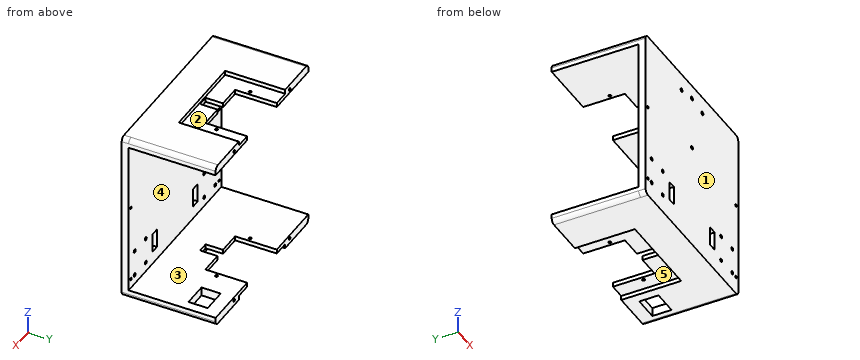
from build123d import *

# Parameters (mm, degrees)
SKETCH_1_W          = 200
SKETCH_1_H          = 200
SKETCH_1_R          = 2.05
SKETCH_1_R_2        = 1.6
SKETCH_1_R_3        = 2.1
SKETCH_1_W_2        = 10
SKETCH_1_H_2        = 22
EXTRUDE_1_DEPTH     = 8
FILLET_1_R          = 5
FILLET_2_R          = 5
FILLET_3_R          = 5
FILLET_4_R          = 5
SKETCH_2_W          = 200
SKETCH_2_H          = 10
EXTRUDE_2_DEPTH     = 100
FILLET_5_R          = 5
FILLET_6_R          = 5
FILLET_7_R          = 5
FILLET_8_R          = 5
SKETCH_3_R          = 1.6
CUT_EXTRUDE_1_DEPTH = 1000
SKETCH_4_W          = 100
SKETCH_4_H          = 69
CUT_EXTRUDE_2_DEPTH = 5
SKETCH_6_R          = 1.6
CUT_EXTRUDE_3_DEPTH = 6
SKETCH_7_W          = 28.1
SKETCH_7_H          = 22.1
CUT_EXTRUDE_4_DEPTH = 100


with BuildPart() as part:
    # 草图1 → 凸台-拉伸1 (new body)
    with BuildSketch(Plane(origin=(0, 0, 0), x_dir=(1, 0, 0), z_dir=(0, 1, 0))):
        Rectangle(SKETCH_1_W, SKETCH_1_H)
        with Locations(Location((-87, 49, 0), (0, 0, 270))):
            Circle(SKETCH_1_R, mode=Mode.SUBTRACT)
        with Locations(Location((-63, 49, 0), (0, 0, 270))):
            Circle(SKETCH_1_R, mode=Mode.SUBTRACT)
        with Locations(Location((-63, 79, 0), (0, 0, 270))):
            Circle(SKETCH_1_R, mode=Mode.SUBTRACT)
        with Locations(Location((-87, 79, 0), (0, 0, 270))):
            Circle(SKETCH_1_R, mode=Mode.SUBTRACT)
        with Locations(Location((87, 49, 0), (0, 0, 90))):
            Circle(SKETCH_1_R, mode=Mode.SUBTRACT)
        with Locations(Location((63, 49, 0), (0, 0, 90))):
            Circle(SKETCH_1_R, mode=Mode.SUBTRACT)
        with Locations(Location((63, 79, 0), (0, 0, 90))):
            Circle(SKETCH_1_R, mode=Mode.SUBTRACT)
        with Locations(Location((87, 79, 0), (0, 0, 90))):
            Circle(SKETCH_1_R, mode=Mode.SUBTRACT)
        with Locations(Location((-95, 79, 0), (0, 0, 270))):
            Circle(SKETCH_1_R_2, mode=Mode.SUBTRACT)
        with Locations(Location((95, 79, 0), (0, 0, 270))):
            Circle(SKETCH_1_R_2, mode=Mode.SUBTRACT)
        with Locations(Location((95, -11, 0), (0, 0, 270))):
            Circle(SKETCH_1_R_2, mode=Mode.SUBTRACT)
        with Locations(Location((-95, -11, 0), (0, 0, 270))):
            Circle(SKETCH_1_R_2, mode=Mode.SUBTRACT)
        with Locations(Location((0, -22, 0), (0, 0, 270))):
            Circle(SKETCH_1_R_3, mode=Mode.SUBTRACT)
        with Locations(Location((0, -84, 0), (0, 0, 270))):
            Circle(SKETCH_1_R_3, mode=Mode.SUBTRACT)
        with Locations(Location((-22.5, -80, 0), (0, 0, 270))):
            Circle(SKETCH_1_R_3, mode=Mode.SUBTRACT)
        with Locations(Location((22.5, -80, 0), (0, 0, 90))):
            Circle(SKETCH_1_R_3, mode=Mode.SUBTRACT)
        with Locations((44, 64)):
            Rectangle(SKETCH_1_W_2, SKETCH_1_H_2, mode=Mode.SUBTRACT)
        with Locations((-44, 64)):
            Rectangle(SKETCH_1_W_2, SKETCH_1_H_2, mode=Mode.SUBTRACT)
    extrude(amount=EXTRUDE_1_DEPTH)

    # 圆角1
    fillet_1_edges = [part.edges().sort_by_distance(p)[0] for p in [
        (-100, 4, 100),
    ]]
    fillet(fillet_1_edges, radius=FILLET_1_R)

    # 圆角2
    fillet_2_edges = [part.edges().sort_by_distance(p)[0] for p in [
        (100, 4, 100),
    ]]
    fillet(fillet_2_edges, radius=FILLET_2_R)

    # 圆角3
    fillet_3_edges = [part.edges().sort_by_distance(p)[0] for p in [
        (100, 4, -100),
    ]]
    fillet(fillet_3_edges, radius=FILLET_3_R)

    # 圆角4
    fillet_4_edges = [part.edges().sort_by_distance(p)[0] for p in [
        (-100, 4, -100),
    ]]
    fillet(fillet_4_edges, radius=FILLET_4_R)

    # 草图2 → 凸台-拉伸2 (add)
    with BuildSketch(Plane(origin=(0, 8, 0), x_dir=(1, 0, 0), z_dir=(0, 1, 0))):
        with Locations((0, -95)):
            Rectangle(SKETCH_2_W, SKETCH_2_H)
        with Locations((0, 95)):
            Rectangle(SKETCH_2_W, SKETCH_2_H)
    extrude(amount=EXTRUDE_2_DEPTH)

    # 圆角5
    fillet_5_edges = [part.edges().sort_by_distance(p)[0] for p in [
        (100, 58, -100),
    ]]
    fillet(fillet_5_edges, radius=FILLET_5_R)

    # 圆角6
    fillet_6_edges = [part.edges().sort_by_distance(p)[0] for p in [
        (-100, 58, -100),
    ]]
    fillet(fillet_6_edges, radius=FILLET_6_R)

    # 圆角7
    fillet_7_edges = [part.edges().sort_by_distance(p)[0] for p in [
        (-100, 58, 100),
    ]]
    fillet(fillet_7_edges, radius=FILLET_7_R)

    # 圆角8
    fillet_8_edges = [part.edges().sort_by_distance(p)[0] for p in [
        (100, 58, 100),
    ]]
    fillet(fillet_8_edges, radius=FILLET_8_R)

    # 草图3 → 切除-拉伸1 (cut)
    with BuildSketch(Plane(origin=(0, 0, -100), x_dir=(-1, 0, 0), z_dir=(0, 0, -1))):
        with Locations((-36.3, 75.05)):
            Circle(SKETCH_3_R)
        with Locations((36.3, 75.05)):
            Circle(SKETCH_3_R)
        Polygon((-32.05, 108), (32.05, 108), (32.05, 60), (6, 60), (6, 40), (-6, 40), (-6, 60), (-32.05, 60), align=None)
    extrude(amount=-CUT_EXTRUDE_1_DEPTH, mode=Mode.SUBTRACT)

    # 草图4 → 切除-拉伸2 (cut)
    with BuildSketch(Plane(origin=(0, 0, -100), x_dir=(-1, 0, 0), z_dir=(0, 0, -1))):
        with Locations((0, 73.5)):
            Rectangle(SKETCH_4_W, SKETCH_4_H)
    cut_extrude_2 = extrude(amount=-CUT_EXTRUDE_2_DEPTH, mode=Mode.SUBTRACT)

    # 镜向1: 切除-拉伸2 across plane
    add(cut_extrude_2.mirror(Plane.XY), mode=Mode.SUBTRACT)

    # 草图6 → 切除-拉伸3 (cut)
    with BuildSketch(Plane(origin=(0, 108, 0), x_dir=(1, 0, 0), z_dir=(0, 1, 0))):
        with Locations(Location((-60, 94, 0), (0, 0, 270))):
            Circle(SKETCH_6_R)
        with Locations(Location((60, 94, 0), (0, 0, 90))):
            Circle(SKETCH_6_R)
    cut_extrude_3 = extrude(amount=-CUT_EXTRUDE_3_DEPTH, mode=Mode.SUBTRACT)

    # 镜向2: 切除-拉伸3 across plane
    add(cut_extrude_3.mirror(Plane.XY), mode=Mode.SUBTRACT)

    # 草图7 → 切除-拉伸4 (cut)
    with BuildSketch(Plane(origin=(0, 0, -100), x_dir=(-1, 0, 0), z_dir=(0, 0, -1))):
        with Locations((-74.95, 81.95)):
            Rectangle(SKETCH_7_W, SKETCH_7_H)
    extrude(amount=-CUT_EXTRUDE_4_DEPTH, mode=Mode.SUBTRACT)


solid = part.part
Could you check a few things on this model? Use its own coordinates, in mm. Face numbers are marked on the shaded views. A direction names the side the tool comes from. Give positions to 0.01 mm unless a question says otherwise; leave off trailing zeros. Order: outer loops, then holes, each group sorted by start corner. A loop starts at its lowest first (then second) coordinate and runs counter-clockwise, first axis right, second up. Notation, with made-up numbers: (37.25, -8.75) -> (96.25, -8.75) arc R30 cw to (96.25, 16.25) -> close; hole circle Ø6 at (87.25, 1). An arc over 180 degrees is marked (long way). Return JSON: item names as keys, results as strings.
1. Imagine slicing it at D-D on y = 98. List the corners of the cut face in (x, z) for me, then the cut area to 3 significant figures.
Answer list:
{"outline": "(-100, -95) arc R5 ccw to (-95, -100) -> (-50, -100) -> (-50, -95) -> (-32.05, -95) -> (-32.05, -90) -> (-100, -90) -> close; (-100, 90) -> (-32.05, 90) -> (-32.05, 95) -> (-50, 95) -> (-50, 100) -> (-95, 100) arc R5 ccw to (-100, 95) -> close; (32.05, -95) -> (50, -95) -> (50, -100) -> (95, -100) arc R5 ccw to (100, -95) -> (100, -90) -> (32.05, -90) -> close; (32.05, 90) -> (100, 90) -> (100, 95) arc R5 ccw to (95, 100) -> (50, 100) -> (50, 95) -> (32.05, 95) -> close", "area": "2,340 mm2"}
2. Imagine slicing it at B-B on y = 33.5. List the corners of the cut face in (x, z) for me.
Answer list:
{"outline": "(-100, -95) arc R5 ccw to (-95, -100) -> (95, -100) arc R5 ccw to (100, -95) -> (100, -90) -> (-100, -90) -> close; (-100, 90) -> (100, 90) -> (100, 95) arc R5 ccw to (95, 100) -> (-95, 100) arc R5 ccw to (-100, 95) -> close"}
3. I need wall thicknesses on line 1 (X direction, y = 105, z = -94); line 2 (Z direction, x = 63, y = 4.25); line 3 (X direction, y = 4.25, z = -49). Which ranges of each line are inside material? Lowest first, please. Write a range as from..to.
Answer list:
{"line 1": "x = -100..-61.6, -58.4..-32.05, 32.05..58.4, 61.6..100", "line 2": "z = -100..-81.05, -76.95..-51.05, -46.95..100", "line 3": "x = -100..-89.05, -84.95..-65.05, -60.95..60.95, 65.05..84.95, 89.05..100"}
4. Imagine slicing it at C-C on y = 80. Give the number of separate pieces and of enclosed holes in the cut face, then the cut area to 3 significant figures.
Answer list:
{"separate pieces": "5", "enclosed holes": "0", "area": "2,060 mm2"}
5. On a 3-axis mill with a long thin cutter (end or side, diameter ignored), from which of +Z, -Z, +X, -X, +Y, -Y can I reach the whole of each face in a straight line? I mean the marked faces 1, 2 and 3. Say none if no direction works.
Answer list:
{"face 1": "+Z, -Z, +X, -X, -Y", "face 2": "+Z, +Y", "face 3": "+X, -X, +Y"}
6. Imagine slicing it at A-A on x = 45. List the corners of the cut face in (y, z) for me.
Answer list:
{"outline": "(0, -100) -> (39, -100) -> (39, -95) -> (108, -95) -> (108, -90) -> (8, -90) -> (8, -75) -> (0, -75) -> close; (0, -53) -> (8, -53) -> (8, 90) -> (108, 90) -> (108, 95) -> (39, 95) -> (39, 100) -> (0, 100) -> close"}
7. For pin 1 Ø1.5 at (x, z) = (16.5, 92) entering from +Y; pin 2 Ø4 at (x, z) = (-2.5, -96.5) entering from +Y; pin 3 Ø4 at (x, z) = (-95, 11) entering from +Y, each with a flat end and sliding along its axis, tell me the tip position at first contact or that it passes through.
Answer list:
{"pin 1": "stops at y = 60", "pin 2": "stops at y = 40", "pin 3": "stops at y = 8"}
8. Thinking about a two-plate mould opening in X: for the marked faces 4 and 5, which applies, pulls with the +X half, pulls with the -X half, needs draft (parallel to the pull), parting line crosses it, or undercut?
Answer list:
{"face 4": "needs draft", "face 5": "undercut"}
